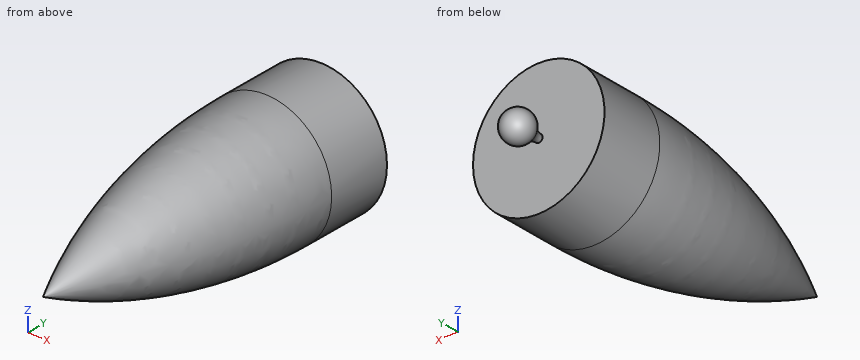
Autodesk Inventor part; units mm, degrees
ref_plane "YZ Plane" through (0, 0, 0) normal (1, 0, 0) x (0, 1, 0)
ref_plane "XZ Plane" through (0, 0, 0) normal (0, 1, 0) x (-1, 0, 0)
ref_plane "XY Plane" through (0, 0, 0) normal (0, 0, 1) x (1, 0, 0)
sketch "Sketch1" plane through (0, 0, 0) normal (0, 0, 1) x (1, 0, 0)
  circle A0 centre (0, 0) radius 3.175
  line L0 (0, 0) -> (3.175, 0)
  line L1 (0, 0) -> (0, -3.175)
  line L2 (0, 0) -> (2.2451, -2.2451)
  line L3 (0, 0) -> (-2.2451, -2.2451)
  line L4 (0, 0) -> (-3.175, 0)
  line L5 (-1.5875, 0) -> (0, 0)
  line L6 (0, 0) -> (1.5875, 0)
  line L7 (0, 0) -> (-0.7938, 0)
  line L8 (0, 0) -> (0.7937, 0)
  line L9 (-0.7938, 0) -> (-0.7938, -7.5506)
  line L10 (-0.7938, -7.5506) -> (0.7937, -7.5506)
  line L11 (0.7937, -7.5506) -> (0.7937, 0)
  arc A1 (-0.7938, -5.1785) -> (-2.2451, -2.2451) centre (-4.4839, -5.1785) ccw
  arc A2 (2.2451, -2.2451) -> (0.7937, -5.1785) centre (4.4839, -5.1785) ccw
  line L12 (0, 3.175) -> (0, -7.5506)
  line L13 (-0.7938, -5.1785) -> (0.7937, -5.1785)
  line L14 (-0.7938, -5.1785) -> (-3.1545, -5.1785)
  line L15 (0.7937, -5.1785) -> (3.1408, -5.1785)
  line L16 (-0.0063, -5.1785) -> (13.6859, -5.1785)
  line L17 (13.6859, -5.1785) -> (13.6859, -18.8349)
  line L18 (13.6859, -18.8349) -> (-0.0064, -18.8349)
  line L19 (-0.0063, -5.1785) -> (-13.6859, -5.1785)
  line L20 (-13.6859, -5.1785) -> (-13.6859, -18.8349)
  line L21 (-13.6859, -18.8349) -> (-0.0064, -18.8349)
  arc A3 (-13.6859, -18.8349) -> (0, -73.864) centre (103.7891, -18.8349) ccw
  arc A4 (0, -73.864) -> (13.6859, -18.8349) centre (-103.7891, -18.8349) ccw
  line L22 (0, -7.5506) -> (0, -73.864)
  line L23 (-13.6859, -18.8349) -> (-10.5109, -18.8349)
  line L24 (13.6859, -18.8349) -> (10.5109, -18.8349)
  line L25 (-13.6859, -5.1785) -> (-13.6859, -8.3535)
  line L26 (-10.5109, -18.8349) -> (-10.5109, -8.3535)
  line L27 (-10.5109, -8.3535) -> (10.5109, -8.3535)
  line L28 (10.5109, -8.3535) -> (10.5109, -18.8349)
  line L29 (0, -73.864) -> (0, -70.689)
  arc A5 (-10.5109, -18.8349) -> (0, -70.689) centre (106.9208, -22.0236) ccw
  arc A6 (0, -70.689) -> (10.5109, -18.8349) centre (-106.9208, -22.0236) ccw
  point P0 (0, 0)
  point P1 (0, -3.175)
  point P2 (1.5373, -5.4355)
  point P3 (0, -5.1785)
  point P4 (0.7937, 0)
  point P5 (0, -8.3535)
  dimension "d0" = 6.35
  dimension "d1" = 45
  dimension "d2" = 45
  dimension "d3" = 7.5506
  dimension "d17" = 13.6564
  dimension "d18" = 5.1785
  dimension "d20" = 13.6922
  dimension "d21" = 13.6796
  dimension "d22" = 117.475
  dimension "d23" = 117.475
  dimension "d27" = 3.175
  dimension "d28" = 3.175
  dimension "d29" = 3.175
  dimension "d30" = 10.4814
  dimension "d31" = 3.175
  dimension "d32" = 117.475
  dimension "d33" = 117.475
revolve "Revolution2" add sketch "Sketch1" angle 360 about axis through (0, 3.175, 0) along (0, -1, 0) contours L0 L12 A0 | A0 L2 L11 L0 | A2 A0 L11 L2 | L2 L11 A0 L1 | L0 L11 L2 | A2 L11 A0 | A0 L11 L13 L12 | L15 L16 L17 L18 L28 L27 L22 L10 L11 | L11 L10 L12 L13 | A4 L22 A6 L18
equation "\"d32\" = d23"
equation "\"d33\" = d23"
properties part number "octopus tentacle end"
The listing builds one solid part. Answer for the finished solid, in the listing's coordinates (mm). Round coordinates to 2 decimals unless told otherwise and drop trailing zeros. Loops run counter-clockwise (first coordinate to the right, second up) from the corner with the lowest first, then second, coordinate; pieces in that order, holes last. Notation, with made-up numbers: (-18, 13) - (39, 13) arc R9 cw to (39, 26) - close; hole circle Ø1 at (89.5, 88.5). An arc over 180 degrees is marked (long way). Use one line per item in the form item = value. Start each with the question number.
1. Given pin 1 Ø3 at (y, z) = (-12, 9.5) entering from -X; pin 2 Ø4 at (y, z) = (-32.5, -8) entering from +X; pin 3 Ø6.5 at (x, z) = (-0.5, -0.5) entering from -Y; pin 4 Ø5 at (x, z) = (4, 7.5) entering from +Y, each flat-ended and moving along its own axis, determine where each tip first touches the part or whether it passes through.
2. Consider line 1 (Z direction, x = 0, y = -16.25); line 2 (Z direction, x = 5.25, y = -49); line 3 (X direction, y = -32.5, z = 5.25). Determine where each line is inside the solid, lowest interval first. Write a range as [from, to].
3. The part is cut by section B-B on y = -10. Determine the outline of the cut face in (x, z), then the cut area to 3 significant figures.
4. The part is cut by section A-A on x = -1.5. Give the number of separate pieces and of enclosed holes in the cut face, then the cut area to 3 significant figures.
Geometry check:
q1.pin_1 = -11.1
q1.pin_2 = 11.44
q1.pin_3 = -73.86
q1.pin_4 = -5.18
q2.line_1 = [-13.69, -10.51], [10.51, 13.69]
q2.line_2 = [-8.21, -5.24], [5.24, 8.21]
q2.line_3 = [-11.77, -8.61], [8.61, 11.77]
q3.outline = circle Ø27.37 at (0, 0); hole circle Ø21.02 at (0, 0)
q3.area = 241 mm^2
q4.separate_pieces = 2
q4.enclosed_holes = 1
q4.area = 439 mm^2
